```python
from build123d import *

# Parameters (mm, degrees)
SKETCH3_W           = 150
SKETCH3_H           = 120
BOSS_EXTRUDE1_DEPTH = 11
SKETCH4_W           = 101
SKETCH4_H           = 81
CUT_EXTRUDE1_DEPTH  = 7
SKETCH5_W           = 90
SKETCH5_H           = 70
CUT_EXTRUDE2_DEPTH  = 5
SKETCH7_R           = 6.5
BOSS_EXTRUDE2_DEPTH = 150


with BuildPart() as part:
    # Sketch3 → Boss-Extrude1 (new body)
    with BuildSketch(Plane(origin=(0, 0, 0), x_dir=(1, 0, 0), z_dir=(0, 1, 0))):
        Rectangle(SKETCH3_W, SKETCH3_H)
    extrude(amount=BOSS_EXTRUDE1_DEPTH)

    # Sketch4 → Cut-Extrude1 (cut)
    with BuildSketch(Plane(origin=(0, 11, 0), x_dir=(1, 0, 0), z_dir=(0, 1, 0))):
        Rectangle(SKETCH4_W, SKETCH4_H)
    extrude(amount=-CUT_EXTRUDE1_DEPTH, mode=Mode.SUBTRACT)

    # Sketch5 → Cut-Extrude2 (cut, through all)
    with BuildSketch(Plane(origin=(0, 4, 0), x_dir=(1, 0, 0), z_dir=(0, 1, 0))):
        Rectangle(SKETCH5_W, SKETCH5_H)
    extrude(amount=-CUT_EXTRUDE2_DEPTH, mode=Mode.SUBTRACT)

    # Sketch7 → Boss-Extrude2 (add)
    with BuildSketch(Plane.ZY.offset(75)):
        with BuildLine():
            Line((41.194351798, 0), (59.397648202, 0))
            ThreePointArc((59.397648202, 0), (50.296, -21.8), (41.194351798, 0))
        make_face()
        with Locations((50.296, -9)):
            Circle(SKETCH7_R, mode=Mode.SUBTRACT)
    boss_extrude2 = extrude(amount=-BOSS_EXTRUDE2_DEPTH)

    # Mirror1: Boss-Extrude2 across plane
    add(boss_extrude2.mirror(Plane.XY))


solid = part.part
```
Geometry: final body of the model. Coordinates: model frame, mm. A direction names the side the tool comes from. Round coordinates to 2 decimals unless told otherwise and drop trailing zeros. Order: outer loops, then holes, each group sorted by start corner. A loop starts at its lowest first (then second) coordinate and runs counter-clockwise, first axis right, second up. Notation, with made-up numbers: (-27, 16) -> (-9, 16) arc R16 cw to (-9, 35) -> close; hole circle Ø3 at (-34.75, -18). An arc over 180 degrees is marked (long way). Write each question's results on one line, items separated by ' | '.
Q1. Section query C-C (z = -6.5). Output: boundary loops of the cut face in (x, y), and give its area (3 significant figures).
Response values:
outline: (-75, 0) -> (-45, 0) -> (-45, 4) -> (-50.5, 4) -> (-50.5, 11) -> (-75, 11) -> close; (45, 0) -> (75, 0) -> (75, 11) -> (50.5, 11) -> (50.5, 4) -> (45, 4) -> close | area: 583 mm²
Q2. Pull-direction query (Y, two-part tool) for faces 1 (the face through (-1.05, -7.048, -56.496)), 2 (the face through (-11, 4, 36)), 3 (the face through (-1.05, -7.048, 56.496)), 4 (the face through (45, 2, 0)); classes: released by +Y, released by -Y, zero draft, split by the parting line, or undercut.
Response values:
face 1: undercut | face 2: released by +Y | face 3: undercut | face 4: zero draft
Q3. Access query for faces 5 (the face through (50.5, 8, 1)), 6 (the face through (-1, 2, -35)), 7 (the face through (-1, 5, -60)), 8 (the face through (-75, 2, 1)), 9 (the face through (-1, 5, 60)). Directions: +Z, -Z, +X, -X, +Y, -Y. A direction counts if a zero-diameter tool reaches every point of the face in a straight line with its end or side. Return the directions, or none.
Response values:
face 5: +Y | face 6: +Y, -Y | face 7: -Z, +X, -X, +Y | face 8: +Z, -Z, -X, +Y, -Y | face 9: +Z, +X, -X, +Y
Q4. Section query B-B (x = 58). Output: boundary loops of the cut face in (y, z), and give its area (3 significant figures).
Response values:
outline: (0, -60) -> (11, -60) -> (11, 60) -> (0, 60) -> (0, 59.4) arc R12.8 ccw (long way) to (0, 41.19) -> (0, -41.19) arc R12.8 ccw (long way) to (0, -59.4) -> close; hole circle Ø13 at (-9, -50.3); hole circle Ø13 at (-9, 50.3) | area: 1,990 mm²
Q5. Section query D-D (y = -18). Output: boundary loops of the cut face in (x, z), and give its area (3 significant figures).
Response values:
outline: (-75, -59.4) -> (75, -59.4) -> (75, -41.19) -> (-75, -41.19) -> close; (-75, 41.19) -> (75, 41.19) -> (75, 59.4) -> (-75, 59.4) -> close | area: 5,460 mm²
Q6. Section query A-A (x = -17.5). Output: boundary loops of the cut face in (y, z), and give its area (3 significant figures).
Response values:
outline: (0, -60) -> (11, -60) -> (11, -40.5) -> (4, -40.5) -> (4, -35) -> (0, -35) -> (0, -41.19) arc R12.8 ccw (long way) to (0, -59.4) -> close; (0, 35) -> (4, 35) -> (4, 40.5) -> (11, 40.5) -> (11, 60) -> (0, 60) -> (0, 59.4) arc R12.8 ccw (long way) to (0, 41.19) -> close; hole circle Ø13 at (-9, -50.3); hole circle Ø13 at (-9, 50.3) | area: 1,140 mm²
Q7. Pin query (flat end, axial travel): pin 1 Ø9 at (x, y) = (16.5, 7.5) entering from -Z; pin 2 Ø1.2 at (x, y) = (-6, 2) entering from +Z; pin 3 Ø0.7 at (x, z) = (-18, -59.5) entering from -Y. Return the tip coordinate at first contact, or that it passes through.
Response values:
pin 1: z = -60 | pin 2: z = 60 | pin 3: y = -18.24
Q8. Ray query, line 1 along Z through (x, y) = (-15, 1); line 2 along Z through (x, y) = (56, -8.5); line 3 along X through (y, z) = (9, 31.5). Return the intervals inside material, ascending.
Response values:
line 1: -60 to -35, 35 to 60 | line 2: -63.09 to -56.78, -43.82 to -37.51, 37.51 to 43.82, 56.78 to 63.09 | line 3: -75 to -50.5, 50.5 to 75
